Autodesk Inventor part; units mm, degrees
ref_plane "YZ Plane" through (0, 0, 0) normal (1, 0, 0) x (0, 1, 0)
ref_plane "XZ Plane" through (0, 0, 0) normal (0, 1, 0) x (-1, 0, 0)
ref_plane "XY Plane" through (0, 0, 0) normal (0, 0, 1) x (1, 0, 0)
sketch "Esboço1" plane through (0, 0, 0) normal (0, 0, 1) x (1, 0, 0)
  line L0 (-3.65, -3.2) -> (3.65, -3.2)
  line L1 (3.65, -3.2) -> (3.65, 3.1)
  line L2 (3.65, 3.1) -> (-3.65, 3.1)
  line L3 (-3.65, 3.1) -> (-3.65, -3.2)
  line L4 (0, 3.1) -> (0, 0)
  dimension "d0" = 7.3
  dimension "d1" = 6.3
extrude "Extrusão1" add sketch "Esboço1" along normal blind 3.5
sketch "Esboço2" plane through (0, 0, 0) normal (1, 0, 0) x (0, 1, 0)
  line L0 (0, 0) -> (0, -6.2)
  line L1 (0, 0) -> (2.1, 0)
  line L2 (-3.2, 0) -> (3.1, 0)
  line L3 (0, -6.2) -> (1.83, -6.2)
  line L4 (1.83, -6.2) -> (2.1, 0)
  dimension "d4" = 6.2
  dimension "d5" = 2.1
  dimension "d6" = 1.83
revolve "Revolução1" add sketch "Esboço2" angle 360 about axis through (0, 0, 0) along (0, 0, -1)
sketch "Esboço3" plane through (0, 0, 3.5) normal (0, 0, 1) x (1, 0, 0)
  line L0 (3.65, 3.1) -> (-3.65, 3.1)
  line L1 (3.65, 3.1) -> (3.15, 3.1)
  line L2 (3.15, 3.1) -> (3.15, 1.4)
  line L3 (3.15, 1.4) -> (3.65, 1.4)
  line L4 (3.65, 1.4) -> (3.65, 3.1)
  line L5 (-3.65, -3.2) -> (3.65, -3.2)
  line L6 (3.65, -1.5) -> (3.15, -1.5)
  line L7 (3.15, -1.5) -> (3.15, -3.2)
  line L8 (3.15, -3.2) -> (3.65, -3.2)
  line L9 (3.65, -3.2) -> (3.65, -1.5)
  line L10 (-3.15, -1.5) -> (-3.65, -1.5)
  line L11 (-3.65, -1.5) -> (-3.65, -3.2)
  line L12 (-3.65, -3.2) -> (-3.15, -3.2)
  line L13 (-3.15, -3.2) -> (-3.15, -1.5)
  line L14 (-3.65, 3.1) -> (-3.65, -3.2)
  line L15 (-3.65, 3.1) -> (-6.7444, 5.2741)
  line L16 (-3.15, 3.1) -> (-3.65, 3.1)
  line L17 (-3.65, 3.1) -> (-3.65, 1.4)
  line L18 (-3.65, 1.4) -> (-3.15, 1.4)
  line L19 (-3.15, 1.4) -> (-3.15, 3.1)
  line L20 (3.65, 3.1) -> (5.0024, 4.4542)
  line L21 (3.65, -3.2) -> (6.7193, -5.088)
  line L22 (-3.65, -3.2) -> (-6.2831, -4.7356)
  point P0 (0, 0)
  point P1 (-3.15, -3.2)
  point P2 (-3.65, 1.4)
  dimension "d8" = 0.5
  dimension "d9" = 1.7
  dimension "d10" = 0.5
  dimension "d11" = 1.7
  dimension "d14" = 0.5
  dimension "d15" = 1.7
  dimension "d19" = 0.5
  dimension "d20" = 1.7
extrude "Extrusão2" add sketch "Esboço3" along normal blind 3
properties part number "pushbottom3.5mm"
Work out the finished part from the listing and answer in its coordinate system (mm). A direction names the side the tool comes from. Coordinates: 2 decimals unless noted, no trailing zeros. Write each loop counter-clockwise with the first axis right and the second up, starting at its lowest first coordinate (ties: lowest second). Pieces come first, ordered by that corner, then holes. Notation, with made-up numbers: (-32, 4) - (27, 4) arc R9 ccw to (27, 15) - close; hole circle Ø2 at (72.5, 51.25). An arc over 180 degrees is marked (long way). One line per question, with ' | ' between items.
1) Find section B-B, the plane x = 0. Determine the outline of the cut face in (y, z), and give its area (3 significant figures).
Checks:
outline: (-3.2, 0) - (-2.1, 0) - (-1.83, -6.2) - (1.83, -6.2) - (2.1, 0) - (3.1, 0) - (3.1, 3.5) - (-3.2, 3.5) - close | area: 46.4 mm2
2) Find section D-D, the plane x = -2.75. Determine the outline of the cut face in (y, z).
Checks:
outline: (-3.2, 0) - (3.1, 0) - (3.1, 3.5) - (-3.2, 3.5) - close
3) The mould has two halves that part along X. Classify faces 1 (the face through (1.92, -0.43, -3.06)), 2 (the face through (0, -3.2, 2)), 3 (the face through (-3.65, 0, 2)), 4 (the face through (-3.15, -2, 5)): +X half, -X half, draft (parallel to the pull), parting line (faces both ways), or undercut.
Checks:
face 1: parting line | face 2: draft | face 3: -X half | face 4: undercut
4) Find section A-A, the plane y = 2.5. Determine the outline of the cut face in (x, z), and give its area (4 significant figures).
Checks:
outline: (-3.65, 0) - (3.65, 0) - (3.65, 6.5) - (3.15, 6.5) - (3.15, 3.5) - (-3.15, 3.5) - (-3.15, 6.5) - (-3.65, 6.5) - close | area: 28.55 mm2
5) Find section C-C, the plane z = -3.25. Determine the outline of the cut face in (x, y), and give its area (3 significant figures).
Checks:
outline: circle Ø3.92 at (0, 0) | area: 12.0 mm2
6) For faces 5 (the face through (0, 3.1, 2)), 6 (the face through (-3.15, 2, 5)), 7 (the face through (-0.9, -2.1, 0)), determine the directions among +Z, -Z, +X, -X, +Y, -Y from which every point of the face is accessible in a straight line to the end or side of a thin tool.
Checks:
face 5: +Z, -Z, +X, -X, +Y | face 6: +Z, +Y, -Y | face 7: -Z
7) Flat-ended cylindrical pins translate along their axes: P1, Ø1.5, axis at x = 3, y = 2, coming from the -Z side; P2, Ø2, axis at y = -1, z = -3, coming from the +X side. Find the tip coordinate at first contact, or state that the pin passes through.
Checks:
P1: z = 0 | P2: x = 1.99
8) Consider probe 1 along Z at (x, y) = (-2, 0.75); probe 2 along Z at (x, y) = (-1.5, -0.5); probe 3 along Y at (x, z) = (1.25, -1.25). Determine where each line is inside the solid, lowest interval first. Write a range as [from, to].
Checks:
probe 1: [0, 3.5] | probe 2: [-6.2, 3.5] | probe 3: [-1.62, 1.62]
